CAD build for the part. Positions are in the model's coordinates, mm. Face numbers are marked on the shaded views. Coordinates: 2 decimals unless noted, no trailing zeros. Write each loop counter-clockwise with the first axis right and the second up, starting at its lowest first coordinate (ties: lowest second). Pieces come first, ordered by that corner, then holes. Notation, with made-up numbers: M 81,46.5 L 120,46.5 A19 cw 120,58.5 Z; hole C -3,86.25 d5. An arc over 180 degrees is marked long. Put each result on its own line as item: value. Start each with the question number.
```python
from build123d import *

# Parameters (mm, degrees)
SKETCH1_R           = 10
BOSS_EXTRUDE1_DEPTH = 20
SKETCH2_W           = 802.5
SKETCH2_H           = 500
BOSS_EXTRUDE3_DEPTH = 20


with BuildPart() as part:
    # Sketch1 → Boss-Extrude1 (new body)
    with BuildSketch(Plane.XY):
        with BuildLine():
            Line((-401.25, -40), (401.25, -40))
            ThreePointArc((401.25, -40), (416.557337295, -36.9551813), (429.534271247, -28.284271247))
            Line((429.534271247, -28.284271247), (629.534271247, 171.715728753))
            ThreePointArc((629.534271247, 171.715728753), (638.2051813, 215.307337295), (601.25, 240))
            Line((601.25, 240), (533.13708499, 240))
            ThreePointArc((533.13708499, 240), (502.522410401, 233.910362601), (476.568542495, 216.568542495))
            Line((476.568542495, 216.568542495), (323.431457505, 63.431457505))
            ThreePointArc((323.431457505, 63.431457505), (297.477589599, 46.089637399), (266.86291501, 40))
            Line((266.86291501, 40), (-266.86291501, 40))
            ThreePointArc((-266.86291501, 40), (-297.477589599, 46.089637399), (-323.431457505, 63.431457505))
            Line((-323.431457505, 63.431457505), (-476.568542495, 216.568542495))
            ThreePointArc((-476.568542495, 216.568542495), (-502.522410401, 233.910362601), (-533.13708499, 240))
            Line((-533.13708499, 240), (-601.25, 240))
            ThreePointArc((-601.25, 240), (-638.2051813, 215.307337295), (-629.534271247, 171.715728753))
            Line((-629.534271247, 171.715728753), (-429.534271247, -28.284271247))
            ThreePointArc((-429.534271247, -28.284271247), (-416.557337295, -36.9551813), (-401.25, -40))
        make_face()
        with Locations((601.25, 200)):
            Circle(SKETCH1_R, mode=Mode.SUBTRACT)
        with Locations((401.25, 0)):
            Circle(SKETCH1_R, mode=Mode.SUBTRACT)
        with Locations((-401.25, 0)):
            Circle(SKETCH1_R, mode=Mode.SUBTRACT)
        with Locations((-601.25, 200)):
            Circle(SKETCH1_R, mode=Mode.SUBTRACT)
    boss_extrude1 = extrude(amount=BOSS_EXTRUDE1_DEPTH)

    # Sketch2 → Boss-Extrude3 (add)
    with BuildSketch(Plane.XZ.offset(40)):
        with Locations((0, -250)):
            Rectangle(SKETCH2_W, SKETCH2_H)
        with BuildLine():
            Line((-330, -460), (-270, -460))
            ThreePointArc((-270, -460), (-262.928932188, -457.071067812), (-260, -450))
            Line((-260, -450), (-260, -50))
            ThreePointArc((-260, -50), (-262.928932188, -42.928932188), (-270, -40))
            Line((-270, -40), (-330, -40))
            ThreePointArc((-330, -40), (-337.071067812, -42.928932188), (-340, -50))
            Line((-340, -50), (-340, -450))
            ThreePointArc((-340, -450), (-337.071067812, -457.071067812), (-330, -460))
        make_face(mode=Mode.SUBTRACT)
        with BuildLine():
            Line((-220, -450), (-220, -50))
            ThreePointArc((-220, -50), (-217.071067812, -42.928932188), (-210, -40))
            Line((-210, -40), (-150, -40))
            ThreePointArc((-150, -40), (-142.928932188, -42.928932188), (-140, -50))
            Line((-140, -50), (-140, -450))
            ThreePointArc((-140, -450), (-142.928932188, -457.071067812), (-150, -460))
            Line((-150, -460), (-210, -460))
            ThreePointArc((-210, -460), (-217.071067812, -457.071067812), (-220, -450))
        make_face(mode=Mode.SUBTRACT)
        with BuildLine():
            Line((-100, -450), (-100, -50))
            ThreePointArc((-100, -50), (-97.071067812, -42.928932188), (-90, -40))
            Line((-90, -40), (-30, -40))
            ThreePointArc((-30, -40), (-22.928932188, -42.928932188), (-20, -50))
            Line((-20, -50), (-20, -450))
            ThreePointArc((-20, -450), (-22.928932188, -457.071067812), (-30, -460))
            Line((-30, -460), (-90, -460))
            ThreePointArc((-90, -460), (-97.071067812, -457.071067812), (-100, -450))
        make_face(mode=Mode.SUBTRACT)
        with BuildLine():
            Line((20, -450), (20, -50))
            ThreePointArc((20, -50), (22.928932188, -42.928932188), (30, -40))
            Line((30, -40), (90, -40))
            ThreePointArc((90, -40), (97.071067812, -42.928932188), (100, -50))
            Line((100, -50), (100, -450))
            ThreePointArc((100, -450), (97.071067812, -457.071067812), (90, -460))
            Line((90, -460), (30, -460))
            ThreePointArc((30, -460), (22.928932188, -457.071067812), (20, -450))
        make_face(mode=Mode.SUBTRACT)
        with BuildLine():
            Line((140, -450), (140, -50))
            ThreePointArc((140, -50), (142.928932188, -42.928932188), (150, -40))
            Line((150, -40), (210, -40))
            ThreePointArc((210, -40), (217.071067812, -42.928932188), (220, -50))
            Line((220, -50), (220, -450))
            ThreePointArc((220, -450), (217.071067812, -457.071067812), (210, -460))
            Line((210, -460), (150, -460))
            ThreePointArc((150, -460), (142.928932188, -457.071067812), (140, -450))
        make_face(mode=Mode.SUBTRACT)
        with BuildLine():
            Line((260, -450), (260, -50))
            ThreePointArc((260, -50), (262.928932188, -42.928932188), (270, -40))
            Line((270, -40), (330, -40))
            ThreePointArc((330, -40), (337.071067812, -42.928932188), (340, -50))
            Line((340, -50), (340, -450))
            ThreePointArc((340, -450), (337.071067812, -457.071067812), (330, -460))
            Line((330, -460), (270, -460))
            ThreePointArc((270, -460), (262.928932188, -457.071067812), (260, -450))
        make_face(mode=Mode.SUBTRACT)
    extrude(amount=-BOSS_EXTRUDE3_DEPTH)

    # Mirror1: Boss-Extrude1 across plane
    add(boss_extrude1.mirror(Plane(origin=(0, 0, -250), x_dir=(1, 0, 0), z_dir=(0, 0, -1))))


solid = part.part
```
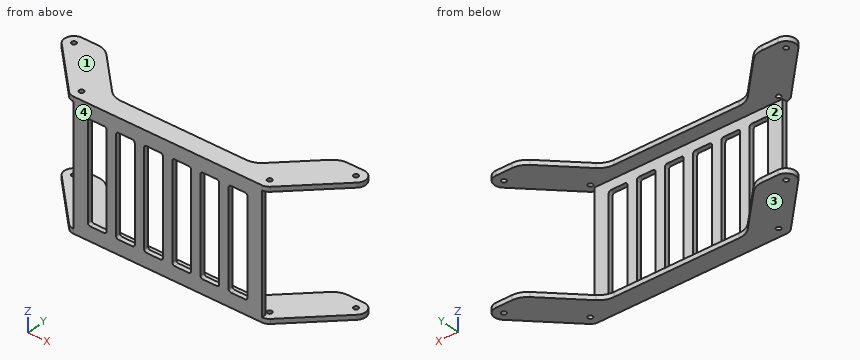
(1) Slice it at B-B, the plane z = -28. Write the cut outline in (x, y).
(2) Drop flat-ended pins along their axis: pin 1 (10 mm diameter, centred on y = -26.5, z = -167, fed in from +X); pin 2 (16 mm diameter, centred on y = -26.5, z = -295, fed in from -X). Give the stop position or say it passes through.
(3) Drill centre lines: line 1 (Z direction, x = -480, y = 206); line 2 (Y direction, x = 224, z = -363.5); line 3 (Y direction, x = 401, z = -510). Where is each one in solid material? Low to high. Write a range as [from, to].
(4) Slice it at A-A, the plane x = -288.5. Write the cut outline in (y, z).
(5) Two-plate mould, pull along Z, no slides. Class the marked faces 1, 2, 3 and 4: +Z half, -Z half, draft (parallel to the pull), parting line (faces both ways), or undercut.
Result set:
1. outline: M -401.25,-40 L 401.25,-40 L 401.25,-20 L -401.25,-20 Z
2. pin 1: stops at x = 401.25
2. pin 2: stops at x = -401.25
3. line 1: z = [-520, -500], [0, 20]
3. line 2: y = [-40, -20]
3. line 3: y = [-40, -10], [10, 141]
4. outline: M -40,-520 L 42.98,-520 L 42.98,-500 L -20,-500 L -20,-460 L -40,-460 Z; M -40,-40 L -20,-40 L -20,0 L 42.98,0 L 42.98,20 L -40,20 Z
5. face 1: +Z half
5. face 2: undercut
5. face 3: -Z half
5. face 4: draft
